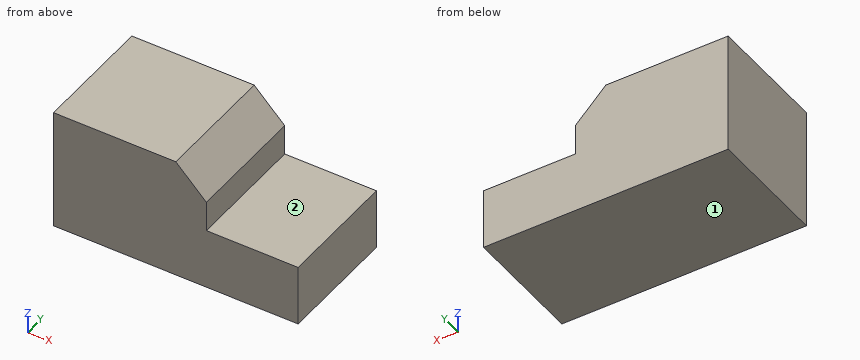
Autodesk Fusion 360 part; units mm, degrees
sketch "Sketch1" plane through (0, 0, 0) normal (0, 0, 1) x (1, 0, 0)
  line L0 (25.4, -12.7) -> (-25.4, -12.7)
  line L1 (-25.4, -12.7) -> (-25.4, 12.7)
  line L2 (-25.4, 12.7) -> (25.4, 12.7)
  line L3 (25.4, 12.7) -> (25.4, -12.7)
  line L4 (25.4, -12.7) -> (-25.4, 12.7) construction
  line L5 (-25.4, -12.7) -> (25.4, 12.7) construction
  dimension "d1" = 50.8
  dimension "d2" = 25.4
extrude "Extrude1" add sketch "Sketch1" along normal blind 25.4
sketch "Sketch2" plane through (0, -12.7, 0) normal (0, -1, 0) x (1, 0, 0)
  line L0 (-25.4, 0) -> (25.4, 0)
  line L1 (25.4, 0) -> (25.4, 25.4)
  line L2 (25.4, 25.4) -> (-25.4, 25.4)
  line L3 (-25.4, 25.4) -> (-25.4, 0)
  line L4 (25.4, 25.4) -> (6.35, 25.4)
  line L5 (6.35, 25.4) -> (6.35, 12.7)
  line L6 (6.35, 12.7) -> (25.4, 12.7)
  line L7 (25.4, 12.7) -> (25.4, 25.4)
  dimension "d5" = 19.05
  dimension "d6" = 12.7
extrude "Extrude2" cut sketch "Sketch2" against normal through all contours L1 L2 L4 L5 L6 L7
chamfer "Chamfer1" distance 6.35 angle 45 1 edges at (6.35, 0, 25.4)
Model file for the job. Use its own axes, mm. Face numbers are marked on the shaded views. A direction names the side the tool comes from. Round coordinates to 2 decimals unless told otherwise and drop trailing zeros. Loops run counter-clockwise (first coordinate to the right, second up) from the corner with the lowest first, then second, coordinate; pieces in that order, holes last.
1. Tool access for the marked faces 1 and 2: list every direction of +Z, -Z, +X, -X, +Y, -Y with a clear straight run to the whole face (end or side of a thin tool).
Check values:
face 1: -Z, +X, -X, +Y, -Y
face 2: +Z, +X, +Y, -Y
2. Band-saw the part on B-B, the plane z = 18.5. List the corners of the cut face in (x, y).
Check values:
outline: (-25.4, -12.7) - (6.35, -12.7) - (6.35, 12.7) - (-25.4, 12.7) - close
3. Drop flat-ended pins along their axis: P1, Ø4, axis at x = 14.5, y = 9, coming from the +Z side; P2, Ø2, axis at y = 9, z = 21.5, coming from the +X side. Give the stop position or say it passes through.
Check values:
P1: stops at z = 12.7
P2: stops at x = 4.9
4. Band-saw the part on C-C, the plane x = 15. List the corners of the cut face in (y, z).
Check values:
outline: (-12.7, 0) - (12.7, 0) - (12.7, 12.7) - (-12.7, 12.7) - close
5. Wall check: probe 1 along X at (y, z) = (-3, 13); probe 2 along Z at (x, y) = (17, 0.5); probe 3 along X at (y, z) = (-9.5, 21.75). Give the ranges that are in metal, low to high.
Check values:
probe 1: x = -25.4 to 6.35
probe 2: z = 0 to 12.7
probe 3: x = -25.4 to 3.65
6. Band-saw the part on A-A, the plane y = 0.5. List the corners of the cut face in (x, z), and give its area (3 significant figures).
Check values:
outline: (-25.4, 0) - (25.4, 0) - (25.4, 12.7) - (6.35, 12.7) - (6.35, 19.05) - (0, 25.4) - (-25.4, 25.4) - close
area: 1,030 mm2
